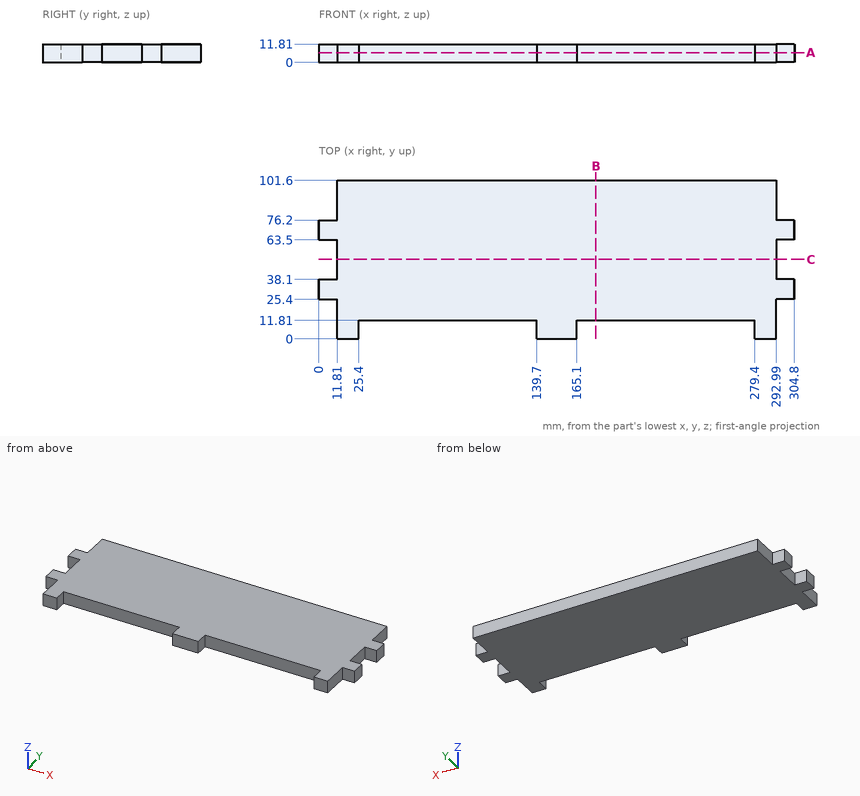
Can you work these out from the drawing? Everything is in mm from the part's minimum corner. Round coordinates to 2 decimals unless told otherwise and drop trailing zeros. Loops run counter-clockwise (first coordinate to the right, second up) from the corner with the lowest first, then second, coordinate; pieces in that order, holes last. Notation, with made-up numbers: (49.5, -36.75) -> (63.5, -36.75) arc R21 ccw to (63.5, -9.75) -> close; hole circle Ø6 at (15, -19.5). An arc over 180 degrees is marked (long way). Answer in a Markdown table with one row per item.
Item 1: Suppose I cut it at A-A, the plane z = 6.25. List the corners of the cut face in (x, y) for me.
Answer block:
| item | result |
|---|---|
| outline | (0, 25.4) -> (11.81, 25.4) -> (11.81, 0) -> (25.4, 0) -> (25.4, 11.81) -> (139.7, 11.81) -> (139.7, 0) -> (165.1, 0) -> (165.1, 11.81) -> (279.4, 11.81) -> (279.4, 0) -> (292.99, 0) -> (292.99, 25.4) -> (304.8, 25.4) -> (304.8, 38.1) -> (292.99, 38.1) -> (292.99, 63.5) -> (304.8, 63.5) -> (304.8, 76.2) -> (292.99, 76.2) -> (292.99, 101.6) -> (11.81, 101.6) -> (11.81, 76.2) -> (0, 76.2) -> (0, 63.5) -> (11.81, 63.5) -> (11.81, 38.1) -> (0, 38.1) -> close |
Item 2: If I drill on probe 1 along X at (y, z) = (11, 11.5); probe 2 along X at (y, z) = (96, 2.75); probe 3 along Y at (x, z) = (79, 9), over which ranges is the centre line in solid material (lowest first)?
Answer block:
| item | result |
|---|---|
| probe 1 | 11.81 to 25.4, 139.7 to 165.1, 279.4 to 292.99 |
| probe 2 | 11.81 to 292.99 |
| probe 3 | 11.81 to 101.6 |
Item 3: Suppose I cut it at C-C, the plane y = 51. List the corners of the cut face in (x, z) for me.
Answer block:
| item | result |
|---|---|
| outline | (11.81, 0) -> (292.99, 0) -> (292.99, 11.81) -> (11.81, 11.81) -> close |
Item 4: Will these pins go through, and if not, where does the flat tip stop? P1, Ø1.5, axis at y = 50.5, z = 8, coming from the -X side; P2, Ø3, axis at x = 241.5, z = 1.5, coming from the -Y side; P3, Ø6, axis at x = 8.5, z = 5, coming from the +Y side.
Answer block:
| item | result |
|---|---|
| P1 | x = 11.81 |
| P2 | y = 11.81 |
| P3 | y = 76.2 |
Item 5: Suppose I cut it at B-B, the plane x = 177.5. List the corners of the cut face in (y, z) for me.
Answer block:
| item | result |
|---|---|
| outline | (11.81, 0) -> (101.6, 0) -> (101.6, 11.81) -> (11.81, 11.81) -> close |
